Check sheet for the drawn part. Datum: minimum x, y, z corner. Units: mm. A direction names the side the tool comes from. Give positions to 0.01 mm unless a question says otherwise; leave off trailing zeros. Write each loop counter-clockwise with the first axis right and the second up, starting at its lowest first coordinate (ties: lowest second). Pieces come first, ordered by that corner, then holes. Notation, with made-up numbers: M 69,76 L 101,76 A16 cw 101,102 Z; hole C -34.75,33 d1. An arc over 180 degrees is marked long. Write item = value, one per line.
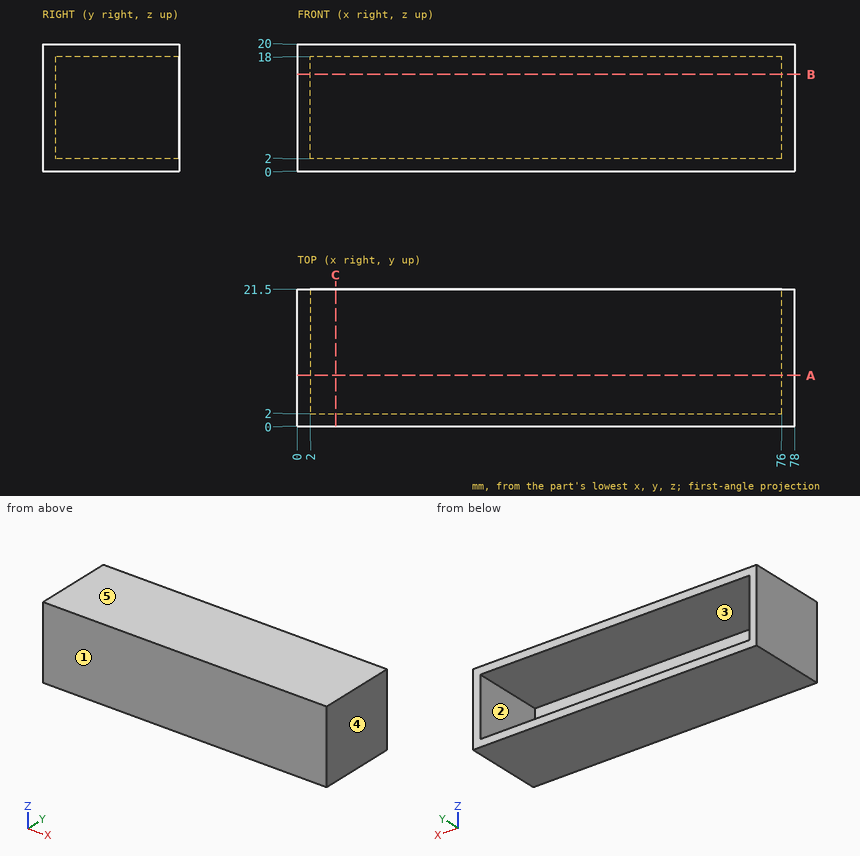
1) Cross-section at C-C on x = 6. Record the boundary of the cut face in (y, z), plus the area to 3 significant figures.
From the geometry:
outline = M 0,0 L 21.5,0 L 21.5,2 L 2,2 L 2,18 L 21.5,18 L 21.5,20 L 0,20 Z
area = 118 mm^2
2) Cross-section at A-A on y = 8. Record the boundary of the cut face in (x, z), plus the area to 3 significant figures.
From the geometry:
outline = M 0,0 L 78,0 L 78,20 L 0,20 Z; hole M 2,2 L 76,2 L 76,18 L 2,18 Z
area = 376 mm^2
3) Draft check along X on the marked faces 3, 4 and 5. Enter one of: +X half, -X half, draft (parallel to the pull), parting line (faces both ways), or undercut.
From the geometry:
face_3 = undercut
face_4 = +X half
face_5 = draft
4) Material ranges on probe 1 along X at (y, z) = (6, 17); probe 2 along Z at (x, y) = (28, 17); probe 3 along Y at (x, z) = (31, 8.5), recorded low to high. Write a range as from..to.
From the geometry:
probe_1 = 0..2, 76..78
probe_2 = 0..2, 18..20
probe_3 = 0..2
5) Tool access check on the marked faces 1 and 2. Record the directions out of +Z, -Z, +X, -X, +Y, -Y that give a thin tool (end or side, any length) a straight path to the whole face; none if there is none.
From the geometry:
face_1 = +Z, -Z, +X, -X, -Y
face_2 = +Y
6) Depth check by flat-ended pin: P1, Ø12, axis at x = 44.5, z = 11, coming from the +Y side. Enter the tip coordinate at first touch or a pass-through.
From the geometry:
P1 = 2
7) Cross-section at B-B on z = 15.25. Record the boundary of the cut face in (x, y).
From the geometry:
outline = M 0,0 L 78,0 L 78,21.5 L 76,21.5 L 76,2 L 2,2 L 2,21.5 L 0,21.5 Z
